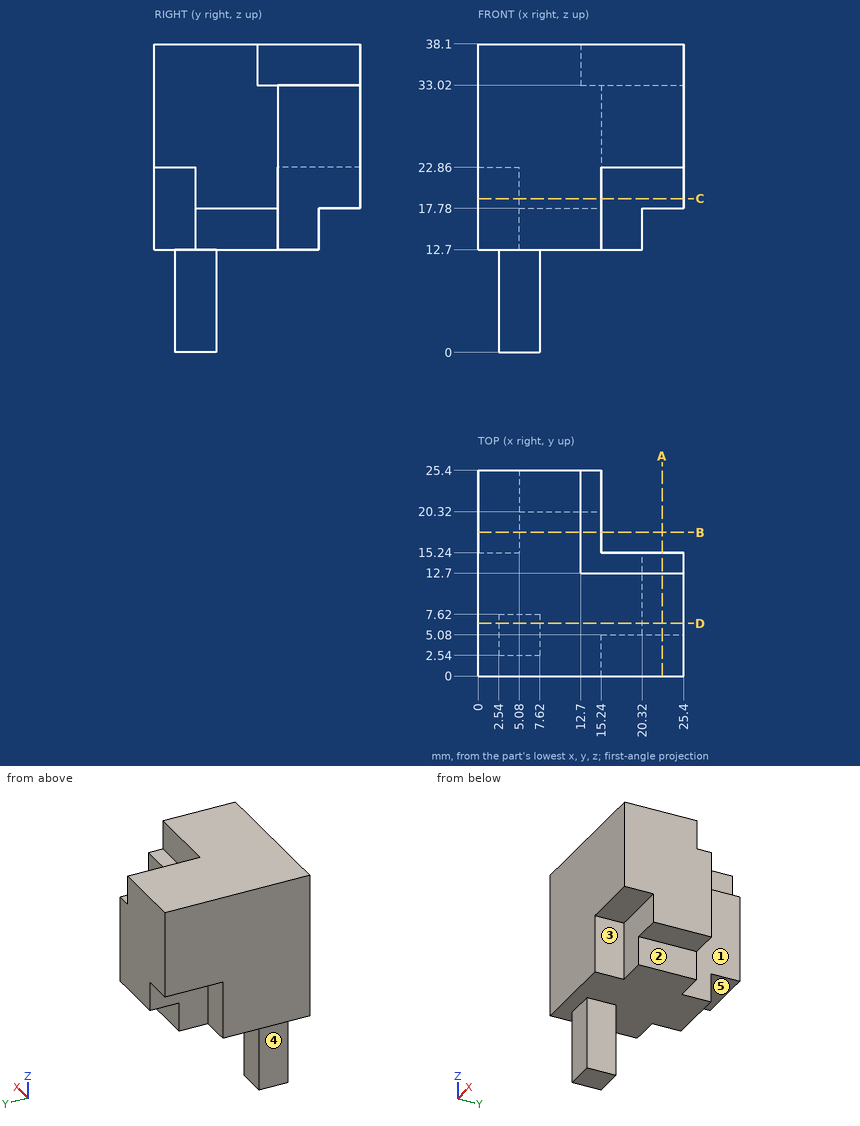
Can you work these out from the drawing? Everything is in mm from the part's minimum corner. A direction names the side the tool comes from. Round coordinates to 2 decimals unless told otherwise and drop trailing zeros. Loops run counter-clockwise (first coordinate to the right, second up) from the corner with the lowest first, then second, coordinate; pieces in that order, holes last. Notation, with made-up numbers: M 35.25,-7 L 48.25,-7 A18 cw 48.25,16 Z; hole C -22.75,-2.75 d3. An arc over 180 degrees is marked long. Write item = value, one per line.
1. Which directions (+Z, -Z, +X, -X, +Y, -Y) give clear straight access to the entire face, cutting with the end or side of a thin tool? Please do the marked faces 1, 2, 3, 4 and 5.
Results below:
face_1 = +Z, -Z, +X, +Y
face_2 = -Z, +X, +Y, -Y
face_3 = -Z, +X, -Y
face_4 = -Z, -X, +Y, -Y
face_5 = -Z, +X, -X, +Y
2. I want a section at C-C, the plane z = 19. Write out the boundary of the cut face in (x, y), and give its area (3 significant figures).
Results below:
outline = M 0,0 L 15.24,0 L 15.24,5.08 L 25.4,5.08 L 25.4,15.24 L 15.24,15.24 L 15.24,25.4 L 5.08,25.4 L 5.08,15.24 L 0,15.24 Z
area = 439 mm²
3. Will these pins go through, and if not, where does the flat tip stop? P1, Ø2.5, axis at x = 5, z = 6.5, coming from the +Y side; P2, Ø3, axis at x = 18.5, z = 19, coming from the -Y side; P3, Ø1.5, axis at x = 4.5, z = 7.5, coming from the -Y side.
Results below:
P1 = 7.62
P2 = 5.08
P3 = 2.54
4. I need wall thicknesses on probe 1 along Y at (x, z) = (5.25, 14.5); probe 2 along Z at (x, y) = (23.75, 11); probe 3 along X at (y, z) = (2, 20). Which ranges of each line are inside material? Lowest first, please.
Results below:
probe_1 = 0 to 20.32
probe_2 = 17.78 to 38.1
probe_3 = 0 to 15.24
5. I want a section at D-D, the plane y = 6.5. Write out the boundary of the cut face in (x, z).
Results below:
outline = M 0,12.7 L 2.54,12.7 L 2.54,0 L 7.62,0 L 7.62,12.7 L 20.32,12.7 L 20.32,17.78 L 25.4,17.78 L 25.4,38.1 L 0,38.1 Z
6. I want a section at B-B, the plane y = 17.75. Write out the boundary of the cut face in (x, z).
Results below:
outline = M 0,22.86 L 5.08,22.86 L 5.08,12.7 L 15.24,12.7 L 15.24,33.02 L 12.7,33.02 L 12.7,38.1 L 0,38.1 Z
7. I want a section at A-A, the plane x = 22.75. Write out the boundary of the cut face in (y, z), and give its area (3 significant figures).
Results below:
outline = M 0,22.86 L 5.08,22.86 L 5.08,17.78 L 15.24,17.78 L 15.24,33.02 L 12.7,33.02 L 12.7,38.1 L 0,38.1 Z
area = 271 mm²
